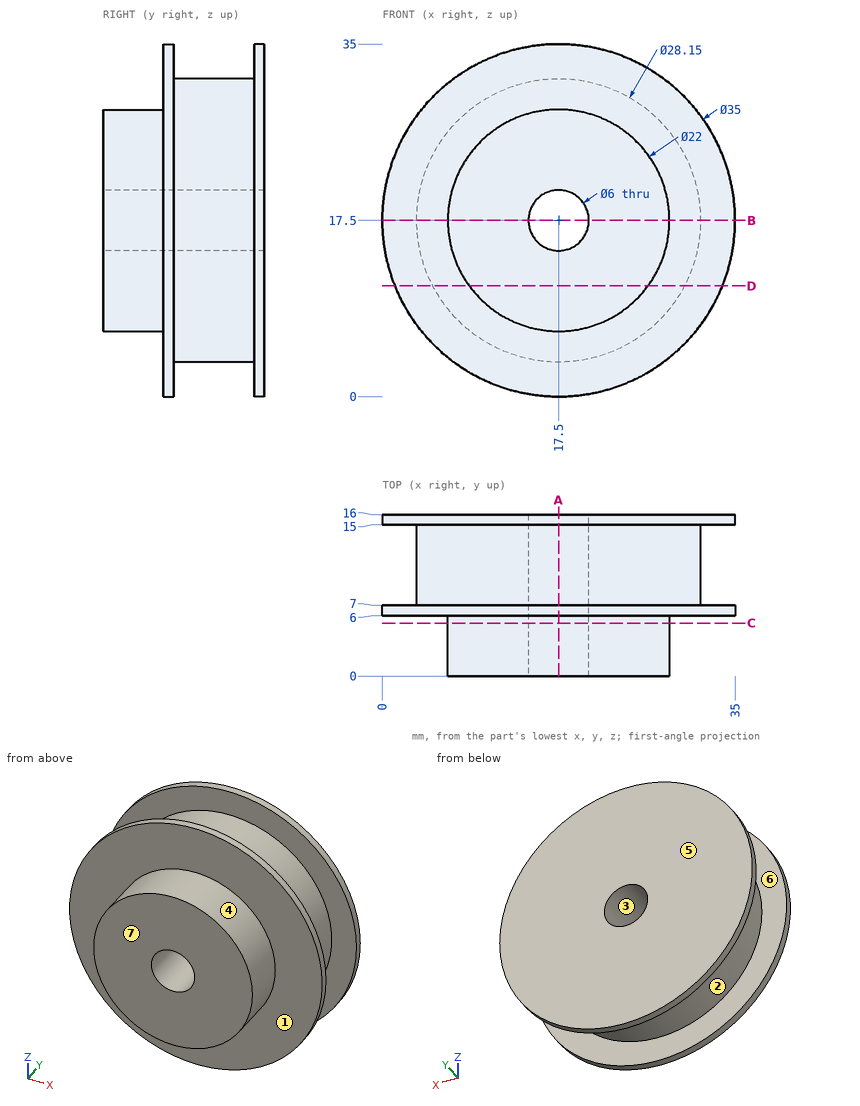
Geometry check sheet. Reference: drawing and pictorial views, mm from the part's lowest x, y, z. A direction names the side the tool comes from. Give positions to 0.01 mm unless a question says otherwise; leave off trailing zeros. Loops run counter-clockwise (first coordinate to the right, second up) from the corner with the lowest first, then second, coordinate; pieces in that order, holes last. Notation, with made-up numbers: (11, 19) - (25, 19) arc R27 cw to (25, 48) - close; hole circle Ø4 at (-9.75, -32.5). An arc over 180 degrees is marked (long way). One line per question, with ' | ' between items. Start each with the question number.
1. Cross-section at C-C, the plane y = 5.25. Enter the section's corners in (x, z).
2. Cross-section at D-D, the plane z = 11. Enter the section's corners in (x, y).
3. Gauge pin test, flat ends, axial feed: pin 1 Ø3 at (y, z) = (7, 13.5) entering from -X; pin 2 Ø9.5 at (x, z) = (17.5, 17.5) entering from -Y; pin 3 Ø5 at (y, z) = (7, 29.5) entering from -X; pin 4 Ø4 at (x, y) = (8, 12) entering from -Z. Record the tip position at first contact, or that the pin passes through.
4. Cross-section at B-B, the plane z = 17.5. Enter the section's corners in (x, y) (3 decimals), plus the area to 3 significant figures.
5. Material ranges on line 1 along Y through (x, z) = (24.5, 3); line 2 along Z through (x, y) = (17.5, 9.5) (3 decimals); line 3 along Z through (x, y) = (17.5, 5), recorded low to high. Write a range as [from, to].
6. Draft check along Y on the marked faces 4, 5, 6 and 7. Enter one of: released by +Y, released by -Y, zero draft, split by the parting line, or undercut.
7. Set-up check for the marked faces 1, 2 and 3: record each of +Z, -Z, +X, -X, +Y, -Y from which the full face is reachable in a straight line by a thin tool's end or side.
8. Cross-section at A-A, the plane x = 17.5. Enter the section's corners in (y, z) (3 decimals), plus the area to 3 significant figures.
Check result:
1) outline: circle Ø22 at (17.5, 17.5); hole circle Ø6 at (17.5, 17.5)
2) outline: (1.25, 6) - (8.63, 6) - (8.63, 0) - (26.37, 0) - (26.37, 6) - (33.75, 6) - (33.75, 7) - (29.98, 7) - (29.98, 15) - (33.75, 15) - (33.75, 16) - (1.25, 16) - (1.25, 15) - (5.02, 15) - (5.02, 7) - (1.25, 7) - close
3) pin 1: stops at x = 0.18 | pin 2: stops at y = 0 | pin 3: stops at x = 2.8 | pin 4: stops at z = 5.59
4) outline: (0, 6) - (6.5, 6) - (6.5, 0) - (14.5, 0) - (14.5, 16) - (0, 16) - (0, 15) - (3.425, 15) - (3.425, 7) - (0, 7) - close; (20.5, 0) - (28.5, 0) - (28.5, 6) - (35, 6) - (35, 7) - (31.575, 7) - (31.575, 15) - (35, 15) - (35, 16) - (20.5, 16) - close | area: 331 mm2
5) line 1: y = [6, 7], [15, 16] | line 2: z = [3.425, 14.5], [20.5, 31.575] | line 3: z = [6.5, 14.5], [20.5, 28.5]
6) face 4: zero draft | face 5: released by +Y | face 6: undercut | face 7: released by -Y
7) face 1: -Y | face 2: none | face 3: +Y, -Y
8) outline: (0, 6.5) - (6, 6.5) - (6, 0) - (7, 0) - (7, 3.425) - (15, 3.425) - (15, 0) - (16, 0) - (16, 14.5) - (0, 14.5) - close; (0, 20.5) - (16, 20.5) - (16, 35) - (15, 35) - (15, 31.575) - (7, 31.575) - (7, 35) - (6, 35) - (6, 28.5) - (0, 28.5) - close | area: 331 mm2
